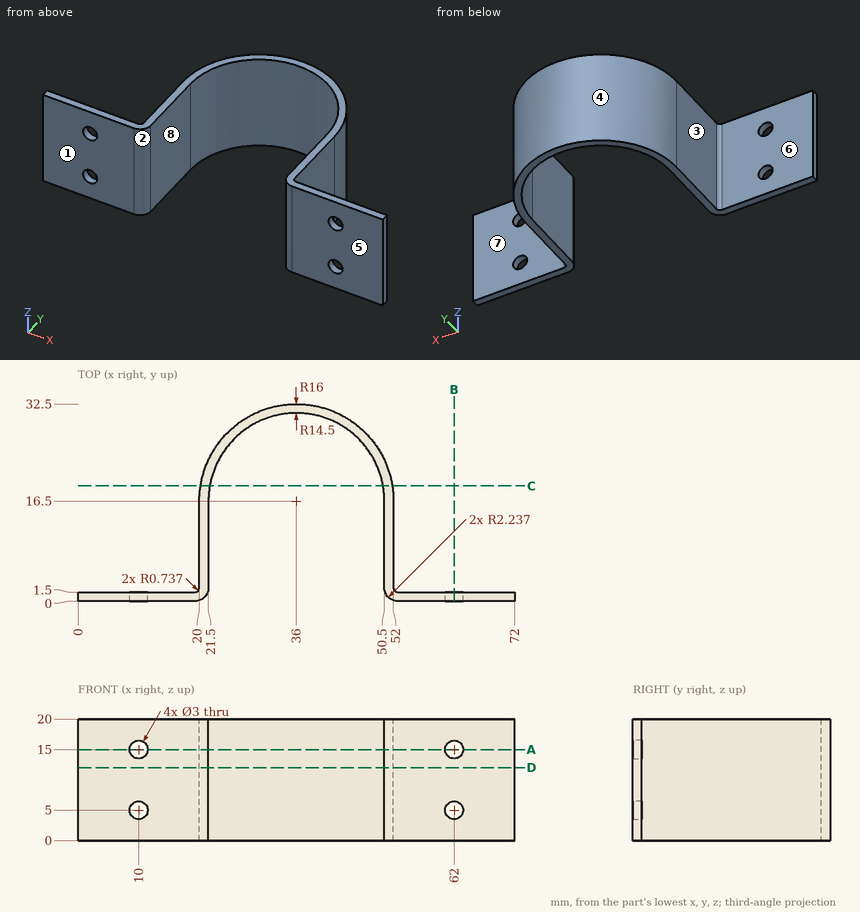
Job drawing, mm, ordinate dimensions from the low corner. One solid piece. A direction names the side the tool comes from. Coordinates: 2 decimals unless noted, no trailing zeros. Order: outer loops, then holes, each group sorted by start corner. A loop starts at its lowest first (then second) coordinate and runs counter-clockwise, first axis right, second up. Notation, with made-up numbers: M -16,-27 L -2,-27 A26 ccw -2,-13 Z; hole C 53,-6.75 d5. An arc over 180 degrees is marked long. One line per question, with ' | ' between items.
Q1. Slice it at C-C (y = 19). Give the cut face in (x, z).
A:
outline: M 20.2,0 L 21.72,0 L 21.72,20 L 20.2,20 Z; M 50.28,0 L 51.8,0 L 51.8,20 L 50.28,20 Z
Q2. Slice it at A-A (z = 15). Give the cut face in (x, y).
A:
outline: M 0,0 L 8.5,0 L 8.5,1.5 L 0,1.5 Z; M 11.5,0 L 19.26,0 A2.24 ccw 21.5,2.24 L 21.5,16.5 A14.5 cw 50.5,16.5 L 50.5,2.24 A2.24 ccw 52.74,0 L 60.5,0 L 60.5,1.5 L 52.74,1.5 A0.74 cw 52,2.24 L 52,16.5 A16 ccw 20,16.5 L 20,2.24 A0.74 cw 19.26,1.5 L 11.5,1.5 Z; M 63.5,0 L 72,0 L 72,1.5 L 63.5,1.5 Z
Q3. Drill centre lines: line 1 (X direction, y = 11, z = 4.75); line 2 (X direction, y = 1.1, z = 5); line 3 (X direction, y = 0.6, z = 15). Where is each one in solid material? Low to high.
A:
line 1: x = 20 to 21.5, 50.5 to 52 | line 2: x = 0 to 8.5, 11.5 to 21.19, 50.81 to 60.5, 63.5 to 72 | line 3: x = 0 to 8.5, 11.5 to 20.79, 51.21 to 60.5, 63.5 to 72
Q4. 3-axis set-ups, long thin cutter, end or side, ignore diameter. For the marked faces 5, 6, 7 and 8: which of +Z, -Z, +X, -X, +Y, -Y reach the whole face in a straight line?
A:
face 5: +Z, -Z, +X, -X, -Y | face 6: +Z, -Z, -X, +Y | face 7: +Z, -Z, +X, +Y | face 8: +Z, -Z, -Y
Q5. Slice it at B-B (x = 62). Give the cut face in (y, z), and give its area (3 significant figures).
A:
outline: M 0,0 L 1.5,0 L 1.5,3.5 L 0,3.5 Z; M 0,6.5 L 1.5,6.5 L 1.5,13.5 L 0,13.5 Z; M 0,16.5 L 1.5,16.5 L 1.5,20 L 0,20 Z | area: 21.0 mm^2
Q6. Two-plate mould, pull along X, no slides. Class the marked faces 1, 2, 3 and 4: +X half, -X half, draft (parallel to the pull), parting line (faces both ways), or undercut.
A:
face 1: draft | face 2: undercut | face 3: -X half | face 4: parting line
Q7. Pin check, flat tips, straight feed: P1, Ø2.5, axis at x = 62, z = 5, coming from the -Y side; P2, Ø7, axis at y = 6, z = 14.5, coming from the +X side; P3, Ø3, axis at x = 62.5, z = 16, coming from the +Y side; P4, Ø7, axis at y = 6.5, z = 6.5, coming from the -X side. Stop position of each tip, or through.
A:
P1: passes through | P2: stops at x = 52 | P3: stops at y = 1.5 | P4: stops at x = 20
Q8. Slice it at D-D (z = 12). Give the cut face in (x, y).
A:
outline: M 0,0 L 19.26,0 A2.24 ccw 21.5,2.24 L 21.5,16.5 A14.5 cw 50.5,16.5 L 50.5,2.24 A2.24 ccw 52.74,0 L 72,0 L 72,1.5 L 52.74,1.5 A0.74 cw 52,2.24 L 52,16.5 A16 ccw 20,16.5 L 20,2.24 A0.74 cw 19.26,1.5 L 0,1.5 Z
